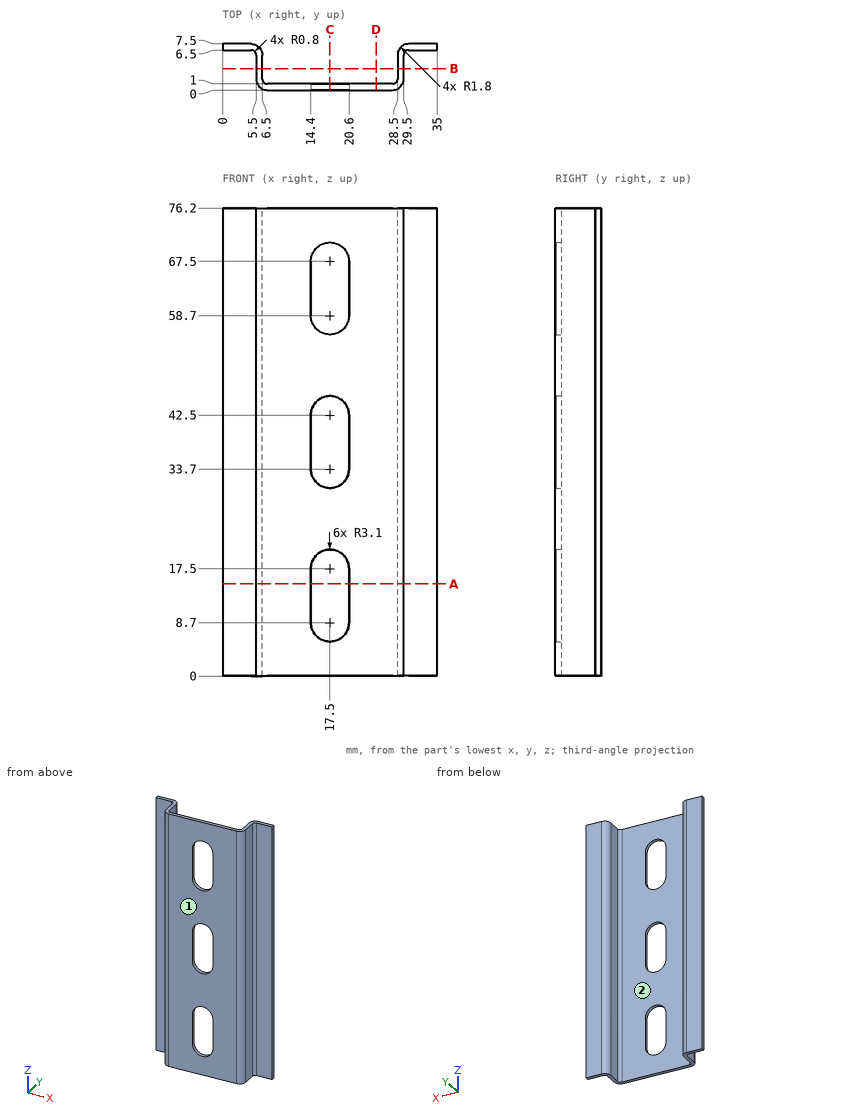
Part print with two shaded views. Sizes in mm from the minimum x, y, z corner. Round coordinates to 2 decimals unless told otherwise and drop trailing zeros. Order: outer loops, then holes, each group sorted by start corner. A loop starts at its lowest first (then second) coordinate and runs counter-clockwise, first axis right, second up.
(1) Pin check, flat tips, straight feed: pin 1 (1.1 mm diameter, centred on y = 0.5, z = 14.5, fed in from -X); pin 2 (6 mm diameter, centred on x = 22, z = 49.5, fed in from +Y); pin 3 (3 mm diameter, centred on y = 2, z = 62.5, fed in from +X). Stop position of each tip, or through.
(2) Drill centre lines: line 1 (X direction, y = 5, z = 73.5); line 2 (Y direction, x = 31, z = 70); line 3 (Y direction, x = 9, z = 12). Where is each one in solid material? Low to high.
(3) Band-saw the part on B-B (y = 3.5). List the corners of the cut face in (x, z).
(4) Pull direction X, two halves, no side cores. Call the marked faces 1 and 2: released by +X, released by -X, zero draft, split by the parting line, or undercut.
(5) Band-saw the part on A-A (z = 15). List the corners of the cut face in (x, y), then the cut area to 3 significant figures.
(6) Band-saw the part on D-D (x = 25). List the corners of the cut face in (y, z), then the cut area to 3 significant figures.
(7) Band-saw the part on C-C (x = 17.5). List the corners of the cut face in (y, z), then the cut area to 3 significant figures.
Verdict:
1. pin 1: stops at x = 5.66
1. pin 2: stops at y = 1
1. pin 3: stops at x = 29.5
2. line 1: x = 5.5 to 6.5, 28.5 to 29.5
2. line 2: y = 6.5 to 7.5
2. line 3: y = 0 to 1
3. outline: (5.5, 0) - (6.5, 0) - (6.5, 76.2) - (5.5, 76.2) - close; (28.5, 0) - (29.5, 0) - (29.5, 76.2) - (28.5, 76.2) - close
4. face 1: zero draft
4. face 2: undercut
5. outline: (0, 6.5) - (4.7, 6.5) arc R0.8 cw to (5.5, 5.7) - (5.5, 1.8) arc R1.8 ccw to (7.3, 0) - (14.4, 0) - (14.4, 1) - (7.3, 1) arc R0.8 cw to (6.5, 1.8) - (6.5, 5.7) arc R1.8 ccw to (4.7, 7.5) - (0, 7.5) - close; (20.6, 0) - (27.7, 0) arc R1.8 ccw to (29.5, 1.8) - (29.5, 5.7) arc R0.8 cw to (30.3, 6.5) - (35, 6.5) - (35, 7.5) - (30.3, 7.5) arc R1.8 ccw to (28.5, 5.7) - (28.5, 1.8) arc R0.8 cw to (27.7, 1) - (20.6, 1) - close
5. area: 39.6 mm2
6. outline: (0, 0) - (1, 0) - (1, 76.2) - (0, 76.2) - close
6. area: 76.2 mm2
7. outline: (0, 0) - (1, 0) - (1, 5.6) - (0, 5.6) - close; (0, 20.6) - (1, 20.6) - (1, 30.6) - (0, 30.6) - close; (0, 45.6) - (1, 45.6) - (1, 55.6) - (0, 55.6) - close; (0, 70.6) - (1, 70.6) - (1, 76.2) - (0, 76.2) - close
7. area: 31.2 mm2
